Here's how the part is built. I have some questions about the finished solid (model axes, mm). A direction names the side the tool comes from. Coordinates: 2 decimals unless noted, no trailing zeros. Write each loop counter-clockwise with the first axis right and the second up, starting at its lowest first coordinate (ties: lowest second). Pieces come first, ordered by that corner, then holes. Notation, with made-up numbers: M 50,30.25 L 86,30.25 A16 cw 86,45.25 Z; hole C -2.5,88 d3. An arc over 180 degrees is marked long. Use a Markdown table: item, result.
```python
from build123d import *

# Parameters (mm, degrees)
F0_W          = 16.298802
F0_H          = 15.749276
F1_DEPTH      = 59.5884
F1_DEPTH_BACK = 59.5884
F2_R          = 5.719222
F3_DEPTH      = 18.542
F4_R          = 1.903741
F5_DEPTH      = 19.05
F6_R          = 1.908705
F7_DEPTH      = 19.05


with BuildPart() as f1:
    # F0 (on Front) → F1 (new body, two sides)
    with BuildSketch(Plane.XZ) as f1_sk:
        Rectangle(F0_W, F0_H)
    extrude(amount=F1_DEPTH)
    extrude(f1_sk.sketch, amount=-F1_DEPTH_BACK)

    # F2 (on face) → F3 (cut)
    with BuildSketch(Plane.YZ.offset(8.149401)):
        Circle(F2_R)
    extrude(amount=-F3_DEPTH, mode=Mode.SUBTRACT)

    # F4 (on face) → F5 (cut)
    with BuildSketch(Plane.XZ.offset(59.5884)):
        Circle(F4_R)
    extrude(amount=-F5_DEPTH, mode=Mode.SUBTRACT)

    # F6 (on face) → F7 (cut)
    with BuildSketch(Plane(origin=(0, 59.5884, 0), x_dir=(-1, 0, 0), z_dir=(0, 1, 0))):
        Circle(F6_R)
    extrude(amount=-F7_DEPTH, mode=Mode.SUBTRACT)


solid = f1.part
```
1. I need wall thicknesses on probe 1 along Z at (x, y) = (0, 51.75); probe 2 along Z at (x, y) = (0, 0); probe 3 along Y at (x, z) = (0, -1.25). Which ranges of each line are inside material? Lowest first, please.
Answers follow:
| item | result |
|---|---|
| probe 1 | z = -7.87 to -1.91, 1.91 to 7.87 |
| probe 2 | z = -7.87 to -5.72, 5.72 to 7.87 |
| probe 3 | y = -40.54 to -5.58, 5.58 to 40.54 |
2. Suppose I cut it at C-C on x = 0. Write out the boundary of the cut face in (y, z).
Answers follow:
| item | result |
|---|---|
| outline | M -59.59,-7.87 L 59.59,-7.87 L 59.59,-1.91 L 40.54,-1.91 L 40.54,1.91 L 59.59,1.91 L 59.59,7.87 L -59.59,7.87 L -59.59,1.9 L -40.54,1.9 L -40.54,-1.9 L -59.59,-1.9 Z; hole C 0,0 d11.44 |
3. Suppose I cut it at A-A on y = 0. Write out the boundary of the cut face in (x, z).
Answers follow:
| item | result |
|---|---|
| outline | M -8.15,-7.87 L 8.15,-7.87 L 8.15,-5.72 L -8.15,-5.72 Z; M -8.15,5.72 L 8.15,5.72 L 8.15,7.87 L -8.15,7.87 Z |
4. We'd pull the mould along X, two halves only. Please class faces 4 (the face through (-0.248, -50.197, 1.888)), 5 (the face through (-2, -59.588, 2)), 6 (the face through (8.149, -1, -7)), 7 (the face through (-8.149, -1, -7)): +X half, -X half, draft (parallel to the pull), parting line (faces both ways), or undercut.
Answers follow:
| item | result |
|---|---|
| face 4 | undercut |
| face 5 | draft |
| face 6 | +X half |
| face 7 | -X half |
5. Which directions (+Z, -Z, +X, -X, +Y, -Y) give clear straight access to the entire face, cutting with the end or side of a thin tool? Please do faces 1 (the face through (0, -40.538, 0)), 2 (the face through (0, -1, 7.875)), 3 (the face through (1.515, 50.197, -1.161)).
Answers follow:
| item | result |
|---|---|
| face 1 | -Y |
| face 2 | +Z, +X, -X, +Y, -Y |
| face 3 | +Y |
6. Suppose I cut it at D-D on y = -42.5. Write out the boundary of the cut face in (x, z).
Answers follow:
| item | result |
|---|---|
| outline | M -8.15,-7.87 L 8.15,-7.87 L 8.15,7.87 L -8.15,7.87 Z; hole C 0,0 d3.81 |
7. Suppose I cut it at B-B on z = 0. Write out the boundary of the cut face in (x, y).
Answers follow:
| item | result |
|---|---|
| outline | M -8.15,-59.59 L -1.9,-59.59 L -1.9,-40.54 L 1.9,-40.54 L 1.9,-59.59 L 8.15,-59.59 L 8.15,-5.72 L -8.15,-5.72 Z; M -8.15,5.72 L 8.15,5.72 L 8.15,59.59 L 1.91,59.59 L 1.91,40.54 L -1.91,40.54 L -1.91,59.59 L -8.15,59.59 Z |
